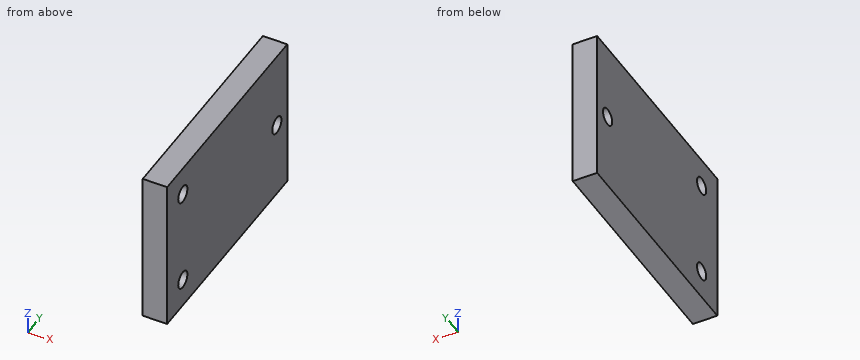
from build123d import *

# Parameters (mm, degrees)
SKETCH1_W           = 55
SKETCH1_H           = 32
BOSS_EXTRUDE1_DEPTH = 46
SKETCH2_W           = 45
SKETCH2_H           = 32
CUT_EXTRUDE1_DEPTH  = 45
SKETCH3_R           = 1.75
CUT_EXTRUDE2_DEPTH  = 47
SKETCH4_R           = 1.75
CUT_EXTRUDE3_DEPTH  = 56
SKETCH7_W           = 32
SKETCH7_H           = 46
CUT_EXTRUDE5_DEPTH  = 50


with BuildPart() as part:
    # Sketch1 → Boss-Extrude1 (new body)
    with BuildSketch(Plane(origin=(0, 0, 0), x_dir=(1, 0, 0), z_dir=(0, 1, 0))):
        with Locations((27.5, 16)):
            Rectangle(SKETCH1_W, SKETCH1_H)
    extrude(amount=BOSS_EXTRUDE1_DEPTH)

    # Sketch2 → Cut-Extrude1 (cut)
    with BuildSketch(Plane.XZ):
        with Locations((27.5, -16)):
            Rectangle(SKETCH2_W, SKETCH2_H)
    extrude(amount=-CUT_EXTRUDE1_DEPTH, mode=Mode.SUBTRACT)

    # Sketch3 → Cut-Extrude2 (cut, through all)
    with BuildSketch(Plane(origin=(0, 46, 0), x_dir=(1, 0, 0), z_dir=(0, 1, 0))):
        with Locations((43.5, 26)):
            Circle(SKETCH3_R)
        with Locations((43.5, 6)):
            Circle(SKETCH3_R)
        with Locations((11.5, 26)):
            Circle(SKETCH3_R)
        with Locations((11.5, 6)):
            Circle(SKETCH3_R)
    extrude(amount=-CUT_EXTRUDE2_DEPTH, mode=Mode.SUBTRACT)

    # Sketch4 → Cut-Extrude3 (cut, through all)
    with BuildSketch(Plane(origin=(55, 0, 0), x_dir=(0, 0, -1), z_dir=(1, 0, 0))):
        with Locations((6, 6)):
            Circle(SKETCH4_R)
        with Locations((26, 6)):
            Circle(SKETCH4_R)
        with Locations((16, 42)):
            Circle(SKETCH4_R)
    extrude(amount=-CUT_EXTRUDE3_DEPTH, mode=Mode.SUBTRACT)

    # Sketch7 → Cut-Extrude5 (cut)
    with BuildSketch(Plane.ZY):
        with Locations((-16, 23)):
            Rectangle(SKETCH7_W, SKETCH7_H)
    extrude(amount=-CUT_EXTRUDE5_DEPTH, mode=Mode.SUBTRACT)


solid = part.part
The model under review builds one solid part; all positions refer to its coordinate system, in mm. Round coordinates to 2 decimals unless told otherwise and drop trailing zeros. Order: outer loops, then holes, each group sorted by start corner. A loop starts at its lowest first (then second) coordinate and runs counter-clockwise, first axis right, second up. Notation, with made-up numbers: (29.5, 77.25) -> (38.5, 77.25) arc R16 ccw to (38.5, 95.25) -> close; hole circle Ø6 at (31.25, 17.5). An arc over 180 degrees is marked (long way). Return JSON: item names as keys, results as strings.
1. Take a section at A-A (z = -5.5). Write out the cut boundary in (x, y), then the cut area to 3 significant figures.
Answer block:
{"outline": "(50, 0) -> (55, 0) -> (55, 4.32) -> (50, 4.32) -> close; (50, 7.68) -> (55, 7.68) -> (55, 46) -> (50, 46) -> close", "area": "213 mm²"}
2. Take a section at C-C (x = 53.5). Write out the cut boundary in (y, z), then the cut area to 3 significant figures.
Answer block:
{"outline": "(0, -32) -> (46, -32) -> (46, 0) -> (0, 0) -> close; hole circle Ø3.5 at (6, -26); hole circle Ø3.5 at (6, -6); hole circle Ø3.5 at (42, -16)", "area": "1,440 mm²"}
3. For L1, parallel to Y at x = 52.45, z = -6; L2, parallel to Y at x = 52.65, z = -16, list the stretches that pass through material, from the lowest coordinate up. Write a range as [from, to].
Answer block:
{"L1": "y = [0, 4.25], [7.75, 46]", "L2": "y = [0, 40.25], [43.75, 46]"}
4. Take a section at B-B (y = 42). Write out the cut boundary in (x, z).
Answer block:
{"outline": "(50, -32) -> (55, -32) -> (55, -17.75) -> (50, -17.75) -> close; (50, -14.25) -> (55, -14.25) -> (55, 0) -> (50, 0) -> close"}
5. Insertion check: P1, Ø1, axis at x = 51.5, z = -15, coming from the -Y side. The pin has a flat end and moves straight along its axis. Give the tip position at first contact, or say it passes through.
Answer block:
{"P1": "stops at y = 0"}
